Design review of the part built by this model. Coordinates are the model's own, in mm. A direction names the side the tool comes from. Coordinates: 2 decimals unless noted, no trailing zeros. Write each loop counter-clockwise with the first axis right and the second up, starting at its lowest first coordinate (ties: lowest second). Pieces come first, ordered by that corner, then holes.
Q1. Machinability: for faces 5 (the flat face through (60.109, 132, 1)), 6 (the flat face through (-59.891, 133, 1)), 7 (the flat face through (-1, 118, -50)), 8 (the cylindrical face through (-10.3, 39.44, 46.37)), 9 (the flat face through (75, 87, 1)), which of the approach directions +Z, -Z, +X, -X, +Y, -Y give a long, thin tool a straight path to every point of the face, cutting with its end or side? Answer none if there is none.
Q2. Insertion check: pin 1 (1.5 mm diameter, centred on x = 49, z = -48.5, fed in from +Y); pin 2 (22.5 mm diameter, centred on y = 122, z = 25, fed in from +X); pin 3 (8 mm diameter, centred on x = -4, z = 22, fed in from +Y). Each pin has a flat end and moves straight along its axis. Give the tip position at first contact, or say it passes through.
Q3. Take a section at A-A (y = 124.5). Give the boundary of the cut face in (x, z), and give its area (3 significant figures).
Q4. Mouldability with a two-part tool opening along Y and no side actions: class faces 1 (the cylindrical face through (1.428, 229.985, 0.7)), 2 (the flat face through (-1, 118, 50)), 3 (the cylindrical face through (-10.73, 121.19, -0.7)), 4 (the flat face through (-34, 80, -34)) as pulls with the +Y half, pulls with the -Y half, needs draft (parallel to the pull), parting line crosses it, or undercut.
Q5. Take a section at C-C (x = -31). Give the boundary of the cut face in (y, z), and give its area (3 significant figures).
Q6. Take a section at D-D (x = -56.5). Give the boundary of the cut face in (y, z), and give its area (3 significant figures).
Q7. For probe 1 along Y at (x, z) = (19, -21); probe 2 along Y at (x, z) = (-37, -38); probe 3 along Z at (x, y) = (60, 106), list the stretches that pass through material, from the lowest coordinate up.
Q8. Take a section at B-B (z = 28.5). Give the boundary of the cut face in (x, y).
```python
from build123d import *

# Parameters (mm, degrees)
SKETCH1_R           = 47.5
BOSS_EXTRUDE1_DEPTH = 80
SKETCH6_W           = 150
SKETCH6_H           = 150
BOSS_EXTRUDE3_DEPTH = 15
SKETCH7_R           = 50
BOSS_EXTRUDE4_DEPTH = 50


with BuildPart() as part:
    # Sketch1 → Boss-Extrude1 (new body)
    with BuildSketch(Plane(origin=(0, 0, 0), x_dir=(1, 0, 0), z_dir=(0, 1, 0))):
        Circle(SKETCH1_R)
    extrude(amount=BOSS_EXTRUDE1_DEPTH)

    # Sketch6 → Boss-Extrude3 (add)
    with BuildSketch(Plane(origin=(0, 80, 0), x_dir=(1, 0, 0), z_dir=(0, 1, 0))):
        Rectangle(SKETCH6_W, SKETCH6_H)
    extrude(amount=BOSS_EXTRUDE3_DEPTH)

    # Sketch7 → Boss-Extrude4 (add, symmetric)
    with BuildSketch(Plane.XY):
        with BuildLine():
            Line((-59.89087621, 95), (60.10912379, 95))
            Line((60.10912379, 95), (60.10912379, 170))
            ThreePointArc((60.10912379, 170), (0.10912379, 230), (-59.89087621, 170))
            Line((-59.89087621, 170), (-59.89087621, 95))
        make_face()
        with Locations((0.10912379, 170)):
            Circle(SKETCH7_R, mode=Mode.SUBTRACT)
    extrude(amount=BOSS_EXTRUDE4_DEPTH, both=True)


solid = part.part
```
Response:
1. face 5: +Z, -Z, +X, +Y
1. face 6: +Z, -Z, -X, +Y
1. face 7: -Z, +X, -X, +Y
1. face 8: -Y
1. face 9: +Z, -Z, +X, +Y, -Y
2. pin 1: stops at y = 205.81
2. pin 2: stops at x = 60.11
2. pin 3: stops at y = 230
3. outline: (-59.89, -50) - (-20.62, -50) - (-20.62, 50) - (-59.89, 50) - close; (20.84, -50) - (60.11, -50) - (60.11, 50) - (20.84, 50) - close
3. area: 7,850 mm2
4. face 1: pulls with the +Y half
4. face 2: needs draft
4. face 3: undercut
4. face 4: pulls with the -Y half
5. outline: (0, -35.99) - (80, -35.99) - (80, -75) - (95, -75) - (95, -50) - (130.86, -50) - (130.86, 50) - (95, 50) - (95, 75) - (80, 75) - (80, 35.99) - (0, 35.99) - close; (209.14, -50) - (221.31, -50) - (221.31, 50) - (209.14, 50) - close
5. area: 12,800 mm2
6. outline: (80, -75) - (95, -75) - (95, -50) - (189.88, -50) - (189.88, 50) - (95, 50) - (95, 75) - (80, 75) - close
6. area: 11,700 mm2
7. probe 1: y = 0 to 123.71, 216.29 to 226.95
7. probe 2: y = 80 to 136.49, 203.51 to 217.15
7. probe 3: z = -50 to 50
8. outline: (-75, 80) - (-38, 80) - (-38, 0) - (38, 0) - (38, 80) - (75, 80) - (75, 95) - (60.11, 95) - (60.11, 170) arc R60 ccw to (-59.89, 170) - (-59.89, 95) - (-75, 95) - close; hole circle Ø100 at (0.11, 170)
